```python
from build123d import *

# Parameters (mm, degrees)
F0_R     = 5.15
F0_R_2   = 13
F1_DEPTH = 8
F3_R     = 13
F4_DEPTH = 230
F5_DEPTH = 25


with BuildPart() as f1:
    # F0 (on Front) → F1 (new body)
    with BuildSketch(Plane.XZ):
        with BuildLine():
            Line((115, 67.621908), (0, 67.621908))
            Line((0, 67.621908), (-115, 67.621908))
            Line((-115, 67.621908), (-115, 37.621908))
            Line((-115, 37.621908), (-73.25, 37.621908))
            ThreePointArc((-73.25, 37.621908), (-65, 45.871908), (-56.75, 37.621908))
            Line((-56.75, 37.621908), (56.75, 37.621908))
            ThreePointArc((56.75, 37.621908), (65, 45.871908), (73.25, 37.621908))
            Line((73.25, 37.621908), (115, 37.621908))
            Line((115, 37.621908), (115, 67.621908))
        make_face()
        with BuildLine():
            Line((-73.25, 37.621908), (-115, 37.621908))
            Line((-115, 37.621908), (-115, 17.621908))
            Line((-115, 17.621908), (-25, -100.378092))
            Line((-25, -100.378092), (0, -100.378092))
            Line((0, -100.378092), (25, -100.378092))
            Line((25, -100.378092), (115, 17.621908))
            Line((115, 17.621908), (115, 37.621908))
            Line((115, 37.621908), (73.25, 37.621908))
            ThreePointArc((73.25, 37.621908), (65, 29.371908), (56.75, 37.621908))
            Line((56.75, 37.621908), (-56.75, 37.621908))
            ThreePointArc((-56.75, 37.621908), (-65, 29.371908), (-73.25, 37.621908))
        make_face()
        with Locations((-30.536113, -35.378092)):
            Circle(F0_R, mode=Mode.SUBTRACT)
        with Locations((0, -59.925269)):
            Circle(F0_R_2, mode=Mode.SUBTRACT)
        with Locations((30.536113, -35.378092)):
            Circle(F0_R, mode=Mode.SUBTRACT)
        with Locations((0, -59.925269)):
            Circle(F0_R_2)
    extrude(amount=F1_DEPTH)

    # F3 (on face) → F4 (cut)
    with BuildSketch(Plane(origin=(0, -8.760227, -1.309225), x_dir=(1, 0, 0), z_dir=(0, -0.989016, -0.147809))):
        with Locations((0, -58.5236)):
            Circle(F3_R)
    extrude(amount=F4_DEPTH, mode=Mode.SUBTRACT)

    # F3 (on face) → F5 (cut)
    with BuildSketch(Plane(origin=(0, -8.760227, -1.309225), x_dir=(1, 0, 0), z_dir=(0, -0.989016, -0.147809))):
        with Locations((0, -58.5236)):
            Circle(F3_R)
    extrude(amount=-F5_DEPTH, mode=Mode.SUBTRACT)


solid = f1.part
```
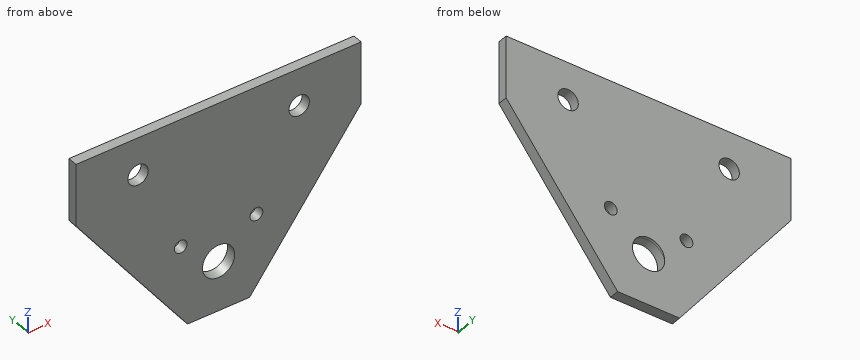
Geometry: final body of the model. Coordinates: model frame, mm. Round coordinates to 2 decimals unless told otherwise and drop trailing zeros. Order: outer loops, then holes, each group sorted by start corner. A loop starts at its lowest first (then second) coordinate and runs counter-clockwise, first axis right, second up. Notation, with made-up numbers: (9, -2) -> (20, -2) arc R21 ccw to (20, 3) -> close; hole circle Ø4 at (59.25, 89.5). An arc over 180 degrees is marked (long way). Use one line per item in the form item = value. Start each with the question number.
1. Cut plane C-C (y = -3.25). Count the separate pieces of the cut face and the enclosed holes in it, then the cut area to 3 significant figures.
2. Cut plane D-D (x = 65). Return the cut outline in (y, z).
3. Line query: probe 1 along Z at (x, y) = (69, -4.25); probe 2 along X at (y, z) = (-5.5, -56); probe 3 along Z at (x, y) = (-4, -4.5). Output: solid intervals per line, ascending.
4. Pin query (flat end, axial travel): pin 1 Ø3 at (y, z) = (-5.5, 16) entering from -X; pin 2 Ø2 at (y, z) = (-4.5, -66.5) entering from -X. Return the tip coordinate at first contact, or that it passes through.
5. Cut plane A-A (x = -10). Return the cut outline in (y, z), then the cut area to 3 significant figures.
6. Cut plane B-B (z = 12). Return the cut outline in (x, y).
Solution:
q1.separate_pieces = 1
q1.enclosed_holes = 5
q1.area = 26,900 mm^2
q2.outline = (-8, -47.93) -> (0, -47.93) -> (0, 29.37) -> (-8, 29.37) -> close; (-8, 45.87) -> (0, 45.87) -> (0, 67.62) -> (-8, 67.62) -> close
q3.probe_1 = -42.69 to 30.41, 44.84 to 67.62
q3.probe_2 = -58.85 to -12.38, 12.38 to 58.85
q3.probe_3 = -100.38 to -72.35, -47.34 to 67.62
q4.pin_1 = -114.91
q4.pin_2 = -51.6
q5.outline = (-8, -100.38) -> (0, -100.38) -> (0, -67.57) -> (-8, -68.77) -> close; (-8, -51.97) -> (0, -50.77) -> (0, 67.62) -> (-8, 67.62) -> close
q5.area = 1,210 mm^2
q6.outline = (-110.71, -8) -> (110.71, -8) -> (110.71, 0) -> (-110.71, 0) -> close
